For this review, take the finished solid that the model builds, in its own axes (mm). A direction names the side the tool comes from. Round coordinates to 2 decimals unless told otherwise and drop trailing zeros. Write each loop counter-clockwise with the first axis right and the second up, starting at its lowest first coordinate (ties: lowest second). Pieces come first, ordered by that corner, then holes. Notation, with made-up numbers: (43.5, 54) -> (97.5, 54) arc R23 cw to (97.5, 65) -> close; hole circle Ø1 at (-37, -1). An arc over 180 degrees is marked (long way). Answer in a Markdown table with one row per item.
from build123d import *

# Parameters (mm, degrees)
SKETCH1_W           = 151
SKETCH1_H           = 95
BOSS_EXTRUDE1_DEPTH = 65
BOSS_EXTRUDE2_DEPTH = 65
CUT_EXTRUDE1_REACH  = 143
SKETCH3_W           = 5
SKETCH3_H           = 7.5
SKETCH3_W_2         = 40


with BuildPart() as part:
    # Sketch1 → Boss-Extrude1 (new body)
    with BuildSketch(Plane.XY):
        Rectangle(SKETCH1_W, SKETCH1_H)
    extrude(amount=-BOSS_EXTRUDE1_DEPTH)

    # Sketch2 → Boss-Extrude2 (add)
    with BuildSketch(Plane.XY):
        Polygon((-65.5, 47.5), (-65.5, 55), (-55.5, 55), (-55.5, 52.5), (-63, 52.5), (-63, 47.5), align=None)
    extrude(amount=-BOSS_EXTRUDE2_DEPTH)

    # Sketch3 → Cut-Extrude1 (cut, up to next)
    with BuildSketch(Plane.ZY.offset(65.5), mode=Mode.PRIVATE) as cut_extrude1_sk1:
        with Locations((-62.5, 51.25)):
            Rectangle(SKETCH3_W, SKETCH3_H)
    cut_extrude1_tool1 = extrude(cut_extrude1_sk1.sketch, amount=-CUT_EXTRUDE1_REACH, mode=Mode.PRIVATE) & part.part
    add(cut_extrude1_tool1.solids().sort_by_distance((-65.5, 51.25, -62.5))[0], mode=Mode.SUBTRACT)
    # Sketch3 → Cut-Extrude1 (cut, up to next)
    with BuildSketch(Plane.ZY.offset(65.5), mode=Mode.PRIVATE) as cut_extrude1_sk2:
        with Locations((-32.5, 51.25)):
            Rectangle(SKETCH3_W_2, SKETCH3_H)
    cut_extrude1_tool2 = extrude(cut_extrude1_sk2.sketch, amount=-CUT_EXTRUDE1_REACH, mode=Mode.PRIVATE) & part.part
    add(cut_extrude1_tool2.solids().sort_by_distance((-65.5, 51.25, -32.5))[0], mode=Mode.SUBTRACT)
    # Sketch3 → Cut-Extrude1 (cut, up to next)
    with BuildSketch(Plane.ZY.offset(65.5), mode=Mode.PRIVATE) as cut_extrude1_sk3:
        with Locations((-2.5, 51.25)):
            Rectangle(SKETCH3_W, SKETCH3_H)
    cut_extrude1_tool3 = extrude(cut_extrude1_sk3.sketch, amount=-CUT_EXTRUDE1_REACH, mode=Mode.PRIVATE) & part.part
    add(cut_extrude1_tool3.solids().sort_by_distance((-65.5, 51.25, -2.5))[0], mode=Mode.SUBTRACT)


solid = part.part
1) Clearance check with flat-ended pins moving along their axes: pin 1 Ø6 at (x, y) = (-59.5, 52.5) entering from +Z; pin 2 Ø0.8 at (y, z) = (54, -7) entering from +X; pin 3 Ø4 at (y, z) = (51.5, -57.5) entering from -X; pin 4 Ø4 at (x, y) = (-59.5, 50) entering from -Z. State where each tip first meets the part, or that it passes through.
Solved:
| item | result |
|---|---|
| pin 1 | z = -5 |
| pin 2 | x = -55.5 |
| pin 3 | x = -65.5 |
| pin 4 | through |
2) Consider section B-B on x = 2. State the section outline as (y, z) points.
Solved:
| item | result |
|---|---|
| outline | (-47.5, -65) -> (47.5, -65) -> (47.5, 0) -> (-47.5, 0) -> close |
3) Mouldability with a two-part tool opening along Z and no side actions: class faces 1 (the flat face through (-1, 1, -65)), 2 (the flat face through (-62, 53, -12.5)), 3 (the flat face through (-61, 55, -56)) as pulls with the +Z half, pulls with the -Z half, needs draft (parallel to the pull), parting line crosses it, or undercut.
Solved:
| item | result |
|---|---|
| face 1 | pulls with the -Z half |
| face 2 | undercut |
| face 3 | needs draft |
4) Consider section C-C on z = -42.5. State the section outline as (x, y) points.
Solved:
| item | result |
|---|---|
| outline | (-75.5, -47.5) -> (75.5, -47.5) -> (75.5, 47.5) -> (-75.5, 47.5) -> close |
5) For faces 4 (the flat face through (-62, 53, -52.5)), 5 (the flat face through (-65.5, 51, -9)), 6 (the flat face through (-62, 53, -60)), 7 (the flat face through (-63, 50, -56)), list the 3-axis set-ups (+Z, -Z, +X, -X, +Y, -Y) from which the entire face can be reached by the end or side of a thin tool; tool diameter is ignored.
Solved:
| item | result |
|---|---|
| face 4 | +X, -X, +Y |
| face 5 | +Z, -Z, -X, +Y |
| face 6 | -Z, +X, -X, +Y |
| face 7 | +Z, -Z, +X |
6) Consider section A-A on z = -10.5. State the section outline as (x, y) points.
Solved:
| item | result |
|---|---|
| outline | (-75.5, -47.5) -> (75.5, -47.5) -> (75.5, 47.5) -> (-63, 47.5) -> (-63, 52.5) -> (-55.5, 52.5) -> (-55.5, 55) -> (-65.5, 55) -> (-65.5, 47.5) -> (-75.5, 47.5) -> close |
7) For line 1 (Y direction, x = 26.5, z = -19.5), list the stretches that pass through material, from the lowest coordinate up. Write a range as [from, to].
Solved:
| item | result |
|---|---|
| line 1 | [-47.5, 47.5] |
